Can you work these out from the model? Positions are in its coordinate system, mm. Face numbers are marked on the shaded views. A direction names the side the tool comes from. Coordinates: 2 decimals unless noted, no trailing zeros. Order: outer loops, then holes, each group sorted by start corner. A loop starts at its lowest first (then second) coordinate and runs counter-clockwise, first axis right, second up. Notation, with made-up numbers: (-24.5, 61.25) - (22.5, 61.25) arc R20 ccw to (22.5, 98.25) - close; hole circle Ø3 at (-9.5, 66.5). An arc over 180 degrees is marked (long way). Use a Markdown table: item, result. Add a question column.
(1) I want a section at C-C (x = -47). List the corners of the cut face in (y, z) for me (3 decimals).
(2) For pin 1 Ø1.6 at (y, z) = (164.29, 0) entering from -X; pin 2 Ø1.5 at (y, z) = (172.5, 1.5) entering from +X; pin 3 Ø3.5 at (y, z) = (169.79, 0) entering from -X, each with a flat end and sliding along its axis, tell me the tip position at first contact or that it passes through.
(3) If I drill on L1, parallel to Y at x = -19.5, z = 2.1; L2, parallel to X at y = 156.5, z = -1; L3, parallel to Y at x = -67.3, z = 0, over which ranges is the centre line in solid material (lowest first)? Write a range as [from, to].
(4) I want a section at A-A (x = -19.5). List the corners of the cut face in (y, z) for me (3 decimals).
(5) I want a section at B-B (z = 2.5). List the corners of the cut face in (x, y) for me.
(6) On a 3-axis mill with a long thin cutter (end or side, diameter ignored), from which of +Z, -Z, +X, -X, +Y, -Y can I reach the whole of each face in a straight line? I mean the marked faces 1 and 2. Say none if no direction works.
```python
from build123d import *

# Parameters (mm, degrees)
SKETCH1_R                = 2.15
BOSS_EXTRUDE1_DEPTH      = 3.175
BOSS_EXTRUDE1_DEPTH_BACK = 3.175
CUT_EXTRUDE1_REACH       = 58
SKETCH2_R                = 1.6
SKETCH3_R                = 3
CUT_EXTRUDE2_DEPTH       = 2.5
SKETCH4_R                = 1.35
CUT_EXTRUDE3_DEPTH       = 5


with BuildPart() as part:
    # Sketch1 → Boss-Extrude1 (new body, two sides)
    with BuildSketch(Plane.XY) as boss_extrude1_sk:
        with BuildLine():
            Line((-70.5, 177.786291501), (-64.5, 177.786291501))
            Line((-64.5, 177.786291501), (-64.5, 165.786291501))
            ThreePointArc((-64.5, 165.786291501), (-65, 165.286291501), (-64.5, 164.786291501))
            Line((-64.5, 164.786291501), (-59.5, 164.786291501))
            Line((-59.5, 164.786291501), (-14.5, 164.786291501))
            Line((-14.5, 164.786291501), (-14.5, 152.786291501))
            Line((-14.5, 152.786291501), (-70.5, 152.786291501))
            Line((-70.5, 152.786291501), (-70.5, 177.786291501))
        make_face()
        with Locations((-65.5, 157.286291501)):
            Circle(SKETCH1_R, mode=Mode.SUBTRACT)
        with Locations((-42.5, 157.286291501)):
            Circle(SKETCH1_R, mode=Mode.SUBTRACT)
        with Locations((-19.5, 157.286291501)):
            Circle(SKETCH1_R, mode=Mode.SUBTRACT)
    extrude(amount=BOSS_EXTRUDE1_DEPTH)
    extrude(boss_extrude1_sk.sketch, amount=-BOSS_EXTRUDE1_DEPTH_BACK)

    # Sketch2 → Cut-Extrude1 (cut, up to next)
    with BuildSketch(Plane.ZY.offset(70.5), mode=Mode.PRIVATE) as cut_extrude1_sk1:
        with Locations((0, 169.786291501)):
            Circle(SKETCH2_R)
    cut_extrude1_tool1 = extrude(cut_extrude1_sk1.sketch, amount=-CUT_EXTRUDE1_REACH, mode=Mode.PRIVATE) & part.part
    add(cut_extrude1_tool1.solids().sort_by_distance((-70.5, 169.786292, 0))[0], mode=Mode.SUBTRACT)

    # Sketch3 → Cut-Extrude2 (cut)
    with BuildSketch(Plane.ZY.offset(70.5)):
        with Locations((0, 169.786291501)):
            Circle(SKETCH3_R)
    extrude(amount=-CUT_EXTRUDE2_DEPTH, mode=Mode.SUBTRACT)

    # Sketch4 → Cut-Extrude3 (cut)
    with BuildSketch(Plane.ZY.offset(70.5)):
        with Locations((0, 175.286291501)):
            Circle(SKETCH4_R)
        with Locations((0, 164.286291501)):
            Circle(SKETCH4_R)
    extrude(amount=-CUT_EXTRUDE3_DEPTH, mode=Mode.SUBTRACT)


solid = part.part
```
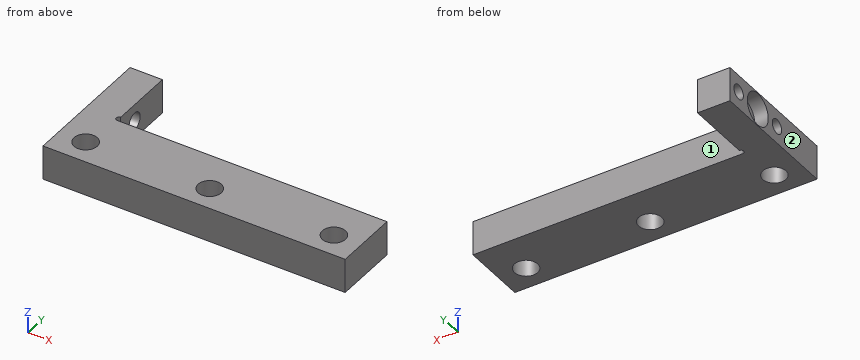
Answers follow:
| question | item | result |
|---|---|---|
| 1 | outline | (152.786, -3.175) - (164.786, -3.175) - (164.786, 3.175) - (152.786, 3.175) - close |
| 2 | pin 1 | stops at x = -65.5 |
| 2 | pin 2 | stops at x = -64.5 |
| 2 | pin 3 | stops at x = -68 |
| 3 | L1 | y = [152.79, 155.14], [159.44, 164.79] |
| 3 | L2 | x = [-70.5, -67.5], [-63.5, -44.5], [-40.5, -21.5], [-17.5, -14.5] |
| 3 | L3 | y = [152.79, 156.11], [158.46, 162.94], [165.64, 168.19], [171.39, 173.94], [176.64, 177.79] |
| 4 | outline | (152.786, -3.175) - (155.136, -3.175) - (155.136, 3.175) - (152.786, 3.175) - close; (159.436, -3.175) - (164.786, -3.175) - (164.786, 3.175) - (159.436, 3.175) - close |
| 5 | outline | (-70.5, 152.79) - (-14.5, 152.79) - (-14.5, 164.79) - (-64.5, 164.79) arc R0.5 cw to (-64.5, 165.79) - (-64.5, 177.79) - (-70.5, 177.79) - (-70.5, 171.44) - (-68, 171.44) - (-68, 168.13) - (-70.5, 168.13) - close; hole circle Ø4.3 at (-65.5, 157.29); hole circle Ø4.3 at (-42.5, 157.29); hole circle Ø4.3 at (-19.5, 157.29) |
| 6 | face 1 | +Z, -Z, +X, +Y |
| 6 | face 2 | +Z, -Z, -X, +Y, -Y |
